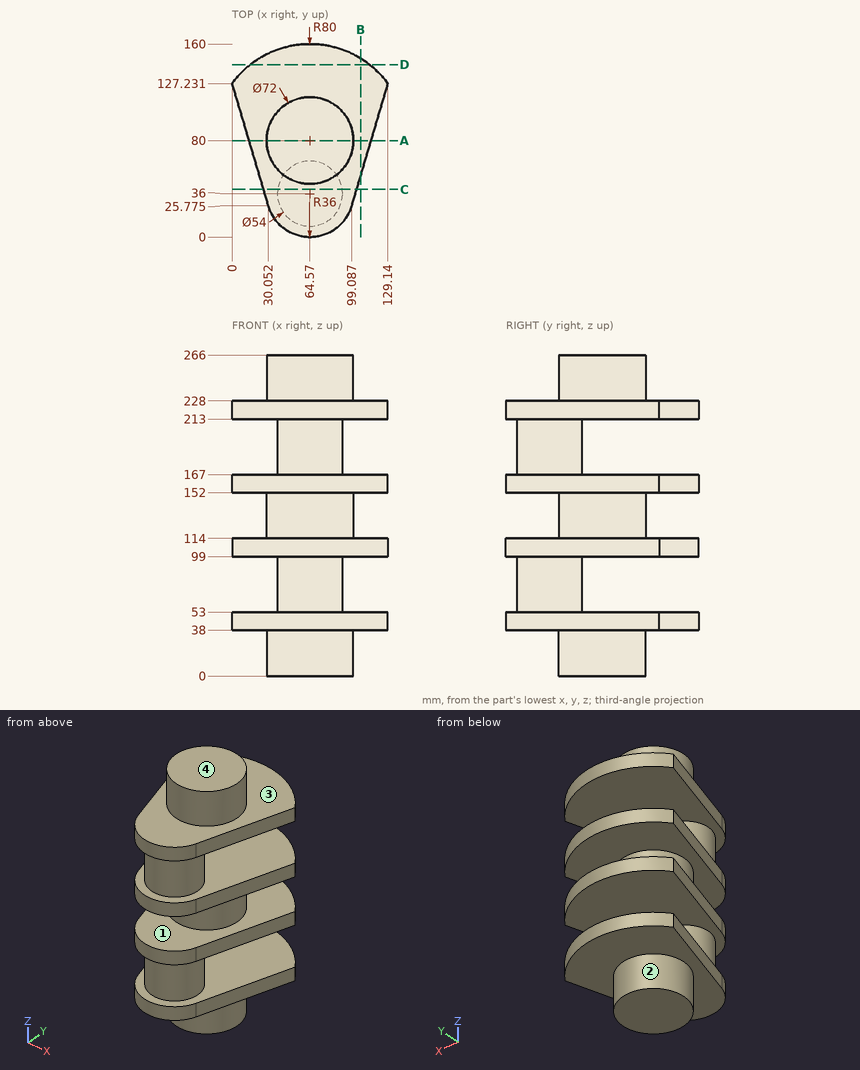
Source: three-view drawing plus pictorial views. Frame: mm from the lowest corner of the part. A direction names the side the tool comes from. Give positions to 0.01 mm unless a question says otherwise; leave off trailing zeros. Loops run counter-clockwise (first coordinate to the right, second up) from the corner with the lowest first, then second, coordinate; pieces in that order, holes last.
1) Line query: L1, parallel to Z at x = 13, y = 85.5; L2, parallel to Z at x = 85.5, y = 76; L3, parallel to X at y = 79.5, z = 241.5. Output: solid intervals per line, ascending.
A:
L1: z = 38 to 53, 99 to 114, 152 to 167, 213 to 228
L2: z = 0 to 53, 99 to 167, 213 to 266
L3: x = 28.57 to 100.57
2) Section query C-C on y = 39.5. Return the cut outline in (x, z), and give its area (3 significant figures).
A:
outline: (25.99, 38) - (103.15, 38) - (103.15, 53) - (91.34, 53) - (91.34, 99) - (103.15, 99) - (103.15, 114) - (25.99, 114) - (25.99, 99) - (37.8, 99) - (37.8, 53) - (25.99, 53) - close; (25.99, 152) - (103.15, 152) - (103.15, 167) - (91.34, 167) - (91.34, 213) - (103.15, 213) - (103.15, 228) - (25.99, 228) - (25.99, 213) - (37.8, 213) - (37.8, 167) - (25.99, 167) - close
area: 9,560 mm2
3) Section query A-A on y = 80. Return the cut outline in (x, z), and give its area (3 significant figures).
A:
outline: (13.99, 38) - (28.57, 38) - (28.57, 0) - (100.57, 0) - (100.57, 38) - (115.15, 38) - (115.15, 53) - (13.99, 53) - close; (13.99, 99) - (115.15, 99) - (115.15, 114) - (100.57, 114) - (100.57, 152) - (115.15, 152) - (115.15, 167) - (13.99, 167) - (13.99, 152) - (28.57, 152) - (28.57, 114) - (13.99, 114) - close; (13.99, 213) - (115.15, 213) - (115.15, 228) - (100.57, 228) - (100.57, 266) - (28.57, 266) - (28.57, 228) - (13.99, 228) - close
area: 14,300 mm2
4) Contact query for flat-ended pins moving along their axis: pin 1 (2 mm diameter, centred on x = 90, z = 178.5, fed in from -Y) (1 decimal); pin 2 (1.5 mm diameter, centred on x = 27, y = 51.5, fed in from +Z); pin 3 (6 mm diameter, centred on x = 62, z = 102.5, fed in from +Y). Output: stop coordinate, or through.
A:
pin 1: stops at y = 24.5
pin 2: stops at z = 228
pin 3: stops at y = 160
5) Section query D-D on y = 143. Return the cut outline in (x, z) (1 decimal), and give its area (3 significant figures).
A:
outline: (15.3, 38) - (113.9, 38) - (113.9, 53) - (15.3, 53) - close; (15.3, 99) - (113.9, 99) - (113.9, 114) - (15.3, 114) - close; (15.3, 152) - (113.9, 152) - (113.9, 167) - (15.3, 167) - close; (15.3, 213) - (113.9, 213) - (113.9, 228) - (15.3, 228) - close
area: 5,920 mm2
6) Section query B-B on x = 106.5. Return the cut outline in (y, z).
A:
outline: (50.8, 38) - (148.13, 38) - (148.13, 53) - (50.8, 53) - close; (50.8, 99) - (148.13, 99) - (148.13, 114) - (50.8, 114) - close; (50.8, 152) - (148.13, 152) - (148.13, 167) - (50.8, 167) - close; (50.8, 213) - (148.13, 213) - (148.13, 228) - (50.8, 228) - close
7) Reachability of the marked faces 1, 2, 3 and 4 from +Z, -Z, +X, -X, +Y, -Y: full face, straight path, thin tool, end or side. Return the list, or none.
A:
face 1: none
face 2: -Z
face 3: +Z
face 4: +Z, +X, -X, +Y, -Y
